Print and shaded views of the part. All mm, measured from the part's lowest x, y and z. A direction names the side the tool comes from. Round coordinates to 2 decimals unless told otherwise and drop trailing zeros. Write each loop counter-clockwise with the first axis right and the second up, starting at its lowest first coordinate (ties: lowest second). Pieces come first, ordered by that corner, then holes. Notation, with made-up numbers: (35, 7) - (64, 7) arc R18 ccw to (64, 38) - close; hole circle Ø6 at (21, -11). An arc over 180 degrees is marked (long way). One line per item, written item: value.
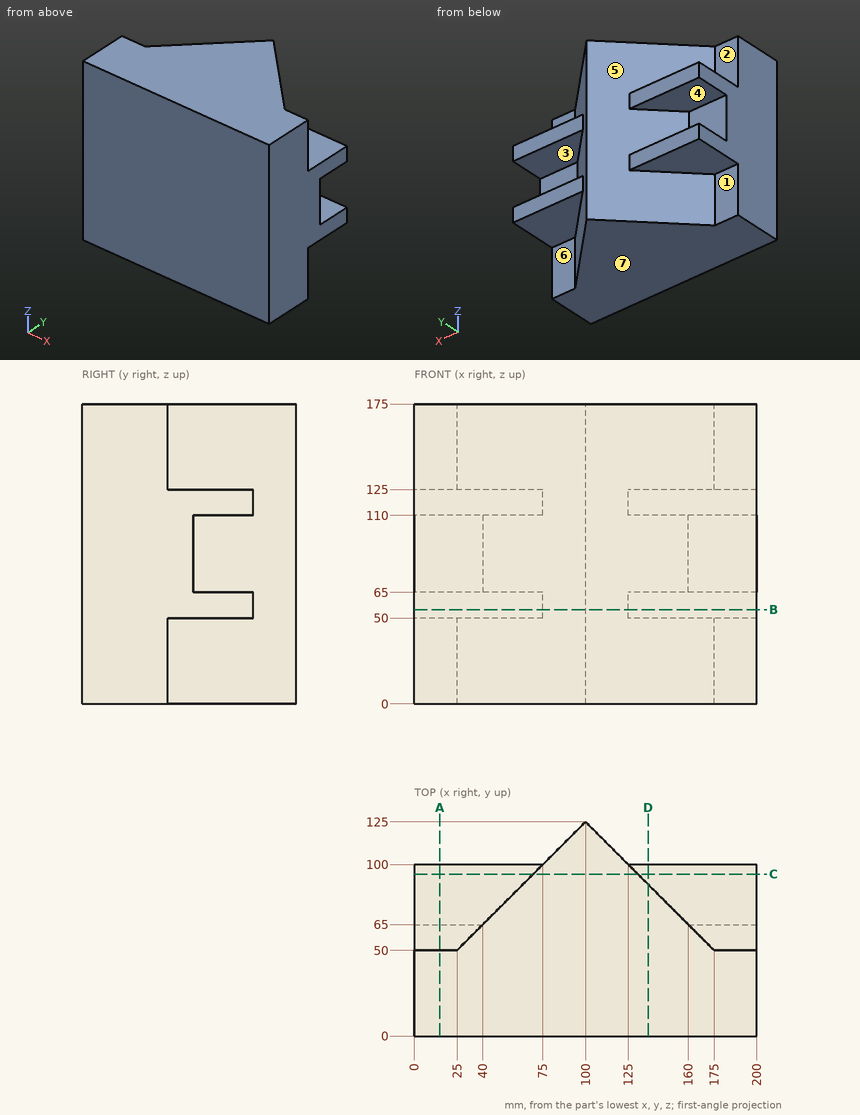
1. Band-saw the part on A-A on x = 15. Write the cut outline in (y, z).
Report:
outline: (0, 0) - (50, 0) - (50, 50) - (100, 50) - (100, 65) - (65, 65) - (65, 110) - (100, 110) - (100, 125) - (50, 125) - (50, 175) - (0, 175) - close
2. Band-saw the part on C-C on y = 94.5. Write the cut outline in (x, z), plus the area to 3 significant figures.
Report:
outline: (0, 50) - (69.5, 50) - (69.5, 0) - (130.5, 0) - (130.5, 50) - (200, 50) - (200, 65) - (130.5, 65) - (130.5, 110) - (200, 110) - (200, 125) - (130.5, 125) - (130.5, 175) - (69.5, 175) - (69.5, 125) - (0, 125) - (0, 110) - (69.5, 110) - (69.5, 65) - (0, 65) - close
area: 14,800 mm²
3. Drop flat-ended pins along their axis: pin 1 (7.5 mm diameter, centred on x = 154, z = 56.5, fed in from +Y); pin 2 (4 mm diameter, centred on x = 135, z = 123, fed in from -Y); pin 3 (10 mm diameter, centred on x = 44.5, z = 19.5, fed in from +Y); pin 4 (7.5 mm diameter, centred on x = 183, z = 32.5, fed in from +Y). Give the stop position or say it passes through.
Report:
pin 1: y = 100
pin 2: y = 0
pin 3: y = 74.5
pin 4: y = 50
4. Wall check: probe 1 along Z at (x, y) = (140, 92); probe 2 along Y at (x, z) = (125, 82); probe 3 along Y at (x, z) = (151.5, 89.5). Give the ranges that are in metal, low to high. Write a range as [from, to].
Report:
probe 1: [50, 65], [110, 125]
probe 2: [0, 100]
probe 3: [0, 73.5]
5. Band-saw the part on D-D on x = 136.5. Write the cut outline in (y, z).
Report:
outline: (0, 0) - (88.5, 0) - (88.5, 50) - (100, 50) - (100, 65) - (88.5, 65) - (88.5, 110) - (100, 110) - (100, 125) - (88.5, 125) - (88.5, 175) - (0, 175) - close
6. Mould opens along Z. For the marked faces 5, 6 and 7 say: released by +Z, released by -Z, zero draft, split by the parting line, or undercut.
Report:
face 5: undercut
face 6: zero draft
face 7: released by -Z
7. Band-saw the part on B-B on z = 55. Write the cut outline in (x, y), plus the area to 3 significant figures.
Report:
outline: (0, 0) - (200, 0) - (200, 100) - (125, 100) - (100, 125) - (75, 100) - (0, 100) - close
area: 20,600 mm²
8. Tool access for the marked faces 1, 2, 3 and 4: list every direction of +Z, -Z, +X, -X, +Y, -Y with a clear straight run to the whole face (end or side of a thin tool).
Report:
face 1: -Z, -X, +Y
face 2: +Z, -X, +Y
face 3: +X, +Y
face 4: -X, +Y
